Source: CAD feature listing. Evaluate the final solid. Frame: model axes, mm. A direction names the side the tool comes from. Give positions to 0.01 mm unless a question says otherwise; leave off trailing zeros. Order: outer loops, then holes, each group sorted by start corner. A loop starts at its lowest first (then second) coordinate and runs counter-clockwise, first axis right, second up.
1) Access query for faces 1 (the face through (96, 55, 61)), 2 (the face through (89, 100, 35)), 3 (the face through (13, 54, 10)), 4 (the face through (162, 45, 61)), 5 (the face through (100, 9, 70)). Directions: +Z, -Z, +X, -X, +Y, -Y. A direction counts if a zero-diameter tool reaches every point of the face in a straight line with its end or side. Return the directions, or none.
2) Draft query along X for faces 6 (the face through (156.15, 19.73, 60.14)), 7 (the face through (153.846, 57.509, 69.72)), 8 (the face through (15.3, 50.4, 20)), 9 (the face through (21.457, 49.54, 35.21)). Return one class per face: released by +X, released by -X, zero draft, split by the parting line, or undercut.
3) Section B-B, the plane x = 77.5. Return loops of the section in (y, z), plus the area to 3 significant figures.
4) Section A-A, the plane z = 28. Return loops of the section in (x, y), plus the area to 3 significant figures.
5) Section D-D, the plane z = 72.5. Return loops of the section in (x, y), plus the area to 3 significant figures.
6) Material intervals for line 1 (Y direction, x = 130, z = 80); line 2 (Y direction, x = 50, z = 20); line 3 (Y direction, x = 157, z = 59), sorted ascending.
7) Section C-C, the plane y = 22. Return loops of the section in (x, z).
8) First-contact query: P1, Ø6, axis at y = 44.5, z = 79, coming from the -X side; P2, Ø20, axis at x = 53, y = 46.5, coming from the +Z side; P3, Ø10.5, axis at x = 10, y = 61, coming from the +Z side; P4, Ø10, axis at x = 50.5, y = 51.5, coming from the +Z side. Flat tips, straight axial feed; report the tip coordinate or a pass-through.
```python
from build123d import *

# Parameters (mm, degrees)
SKETCH1_W                  = 180
SKETCH1_H                  = 100
BOSS_EXTRUDE2_DEPTH        = 70
CUT_EXTRUDE1_DEPTH         = 70
SKETCH3_R                  = 5
CUT_EXTRUDE2_DEPTH         = 70
SKETCH4_R                  = 5
CUT_EXTRUDE3_DEPTH         = 50
SKETCH5_R                  = 10
CUT_EXTRUDE4_DEPTH         = 106
SKETCH6_R                  = 15
CUT_EXTRUDE5_DEPTH         = 40
SKETCH8_R                  = 15
SKETCH8_R_2                = 12.5
BOSS_EXTRUDE3_DEPTH        = 40
SKETCH10_R                 = 12.5
BOSS_EXTRUDE4_DEPTH        = 65
F_25_0MM_DOWEL_HOLE2_D     = 25
F_25_0MM_DOWEL_HOLE2_DEPTH = 20
F_25_0MM_DOWEL_HOLE2_TIP   = 7.510757738
SKETCH12_R                 = 10
SKETCH12_R_2               = 12.5
CUT_EXTRUDE6_DEPTH         = 20
SKETCH13_R                 = 25
SKETCH13_R_2               = 12.5
BOSS_EXTRUDE5_DEPTH        = 40
SKETCH14_R                 = 20
SKETCH14_R_2               = 10
CUT_EXTRUDE7_DEPTH         = 20
BOSS_EXTRUDE10_DEPTH       = 30
BOSS_EXTRUDE13_DEPTH       = 30
CUT_EXTRUDE8_DEPTH         = 5


with BuildPart() as part:
    # Sketch1 → Boss-Extrude2 (new body)
    with BuildSketch(Plane.XY):
        with Locations((90, 50)):
            Rectangle(SKETCH1_W, SKETCH1_H)
    extrude(amount=BOSS_EXTRUDE2_DEPTH)

    # Sketch2 → Cut-Extrude1 (cut)
    with BuildSketch(Plane.XY.offset(70)):
        with BuildLine():
            Line((50, 100), (0, 100))
            Line((0, 100), (0, 50))
            ThreePointArc((0, 50), (14.644660941, 85.355339059), (50, 100))
        make_face()
        with BuildLine():
            ThreePointArc((50, 0), (14.644660941, 14.644660941), (0, 50))
            Line((0, 50), (0, 0))
            Line((0, 0), (50, 0))
        make_face()
        with BuildLine():
            Line((180, 0), (180, 50))
            ThreePointArc((180, 50), (165.355339059, 14.644660941), (130, 0))
            Line((130, 0), (180, 0))
        make_face()
        with BuildLine():
            Line((180, 100), (130, 100))
            ThreePointArc((130, 100), (165.355339059, 85.355339059), (180, 50))
            Line((180, 50), (180, 100))
        make_face()
    extrude(amount=-CUT_EXTRUDE1_DEPTH, mode=Mode.SUBTRACT)

    # Sketch3 → Cut-Extrude2 (cut)
    with BuildSketch(Plane.XY.offset(70)):
        with Locations((10, 50)):
            Circle(SKETCH3_R)
    extrude(amount=-CUT_EXTRUDE2_DEPTH, mode=Mode.SUBTRACT)

    # Sketch4 → Cut-Extrude3 (cut)
    with BuildSketch(Plane.XY.offset(70)):
        with BuildLine():
            ThreePointArc((10, 20), (21.458980338, 50), (10, 80))
            ThreePointArc((10, 80), (0, 50), (10, 20))
        make_face()
        with Locations((10, 50)):
            Circle(SKETCH4_R, mode=Mode.SUBTRACT)
    extrude(amount=-CUT_EXTRUDE3_DEPTH, mode=Mode.SUBTRACT)

    # Sketch5 → Cut-Extrude4 (cut)
    with BuildSketch(Plane.XY.offset(70)):
        with Locations((50, 50)):
            Circle(SKETCH5_R)
    extrude(amount=-CUT_EXTRUDE4_DEPTH, mode=Mode.SUBTRACT)

    # Sketch6 → Cut-Extrude5 (cut)
    with BuildSketch(Plane.XY.offset(70)):
        with Locations((130, 50)):
            Circle(SKETCH6_R)
    extrude(amount=-CUT_EXTRUDE5_DEPTH, mode=Mode.SUBTRACT)

    # Sketch8 → Boss-Extrude3 (add)
    with BuildSketch(Plane.XY.offset(70)):
        with Locations((130, 50)):
            Circle(SKETCH8_R)
        with Locations((130, 50)):
            Circle(SKETCH8_R_2, mode=Mode.SUBTRACT)
    extrude(amount=-BOSS_EXTRUDE3_DEPTH)

    # Sketch10 → Boss-Extrude4 (add)
    with BuildSketch(Plane.XY.offset(70)):
        with Locations((130, 50)):
            Circle(SKETCH10_R)
    extrude(amount=-BOSS_EXTRUDE4_DEPTH)

    # Ø25.0mm Dowel Hole2
    with Locations(Plane(origin=(130, 50, 70), x_dir=(1, 0, 0), z_dir=(0, 0, 1))):
        with Locations((0, 0)):
            Hole(F_25_0MM_DOWEL_HOLE2_D / 2, depth=F_25_0MM_DOWEL_HOLE2_DEPTH)
            with Locations((0, 0, -(F_25_0MM_DOWEL_HOLE2_DEPTH + F_25_0MM_DOWEL_HOLE2_TIP / 2))):  # 118° drill point
                Cone(0, F_25_0MM_DOWEL_HOLE2_D / 2, F_25_0MM_DOWEL_HOLE2_TIP, mode=Mode.SUBTRACT)

    # Sketch12 → Cut-Extrude6 (cut)
    with BuildSketch(Plane.XY.offset(70)):
        with BuildLine():
            ThreePointArc((130, 10), (170, 50), (130, 90))
            Line((130, 90), (20, 90))
            ThreePointArc((20, 90), (14.644660941, 85.355339059), (10, 80))
            ThreePointArc((10, 80), (21.458980338, 50), (10, 20))
            ThreePointArc((10, 20), (14.644660941, 14.644660941), (20, 10))
            Line((20, 10), (130, 10))
        make_face()
        with Locations((50, 50)):
            Circle(SKETCH12_R, mode=Mode.SUBTRACT)
        with Locations((130, 50)):
            Circle(SKETCH12_R_2, mode=Mode.SUBTRACT)
    extrude(amount=-CUT_EXTRUDE6_DEPTH, mode=Mode.SUBTRACT)

    # Sketch13 → Boss-Extrude5 (add)
    with BuildSketch(Plane.XY.offset(50)):
        with Locations((130, 50)):
            Circle(SKETCH13_R)
        with Locations((130, 50)):
            Circle(SKETCH13_R_2, mode=Mode.SUBTRACT)
    extrude(amount=BOSS_EXTRUDE5_DEPTH)

    # Sketch14 → Cut-Extrude7 (cut)
    with BuildSketch(Plane.XY.offset(50)):
        with Locations((50, 50)):
            Circle(SKETCH14_R)
        with Locations((50, 50)):
            Circle(SKETCH14_R_2, mode=Mode.SUBTRACT)
    extrude(amount=-CUT_EXTRUDE7_DEPTH, mode=Mode.SUBTRACT)

    # Sketch15 → Boss-Extrude10 (add)
    with BuildSketch(Plane.XY.offset(50)):
        with BuildLine():
            Line((105.505102572, 45), (105.505102572, 55))
            ThreePointArc((105.505102572, 55), (105, 50), (105.505102572, 45))
        make_face()
        with BuildLine():
            ThreePointArc((105.505102572, 45), (105, 50), (105.505102572, 55))
            Line((105.505102572, 55), (80.505102572, 55))
            Line((80.505102572, 55), (80.505102572, 45))
            Line((80.505102572, 45), (105.505102572, 45))
        make_face()
    extrude(amount=BOSS_EXTRUDE10_DEPTH)

    # Sketch16 → Boss-Extrude13 (add)
    with BuildSketch(Plane.XY.offset(50)):
        with BuildLine():
            Line((169.686269666, 55), (154.494897428, 55))
            ThreePointArc((154.494897428, 55), (155, 50), (154.494897428, 45))
            Line((154.494897428, 45), (169.686269666, 45))
            ThreePointArc((169.686269666, 45), (169.921490369, 47.495083498), (170, 50))
            ThreePointArc((170, 50), (169.921490369, 52.504916502), (169.686269666, 55))
        make_face()
    extrude(amount=BOSS_EXTRUDE13_DEPTH)

    # Sketch18 → Cut-Extrude8 (cut, symmetric)
    with BuildSketch(Plane(origin=(0, 50, 0), x_dir=(1, 0, 0), z_dir=(0, 1, 0))):
        Polygon((155.156999003, -80), (170.098617307, -70), (170.098617307, -80), align=None)
        Polygon((104.578940911, -80), (80.505102572, -50), (80.505102572, -80), align=None)
    extrude(amount=CUT_EXTRUDE8_DEPTH, both=True, mode=Mode.SUBTRACT)


solid = part.part
```
From the geometry:
1. face 1: +Z, -X
1. face 2: +Z, -Z, +X, -X, +Y
1. face 3: +Z, -Z
1. face 4: +Z
1. face 5: +Z, +X
2. face 6: undercut
2. face 7: undercut
2. face 8: zero draft
2. face 9: released by -X
3. outline: (0, 0) - (100, 0) - (100, 70) - (90, 70) - (90, 50) - (10, 50) - (10, 70) - (0, 70) - close
3. area: 5,400 mm2
4. outline: (10, 20) arc R50 ccw to (50, 0) - (130, 0) arc R50 ccw to (130, 100) - (50, 100) arc R50 ccw to (10, 80) arc R45 cw to start; hole circle Ø20 at (50, 50)
4. area: 14,700 mm2
5. outline: (98.56, 45) - (105.51, 45) arc R25 ccw to (154.49, 45) - (166.36, 45) - (166.36, 55) - (154.49, 55) arc R25 ccw to (105.51, 55) - (98.56, 55) - close; hole circle Ø25 at (130, 50)
5. area: 1,650 mm2
6. line 1: y = 25 to 37.5, 62.5 to 75
6. line 2: y = 0 to 40, 60 to 100
6. line 3: y = 7.92 to 20.49, 45 to 55, 79.51 to 92.08
7. outline: (8.58, 0) - (171.42, 0) - (171.42, 70) - (158.57, 70) - (158.57, 50) - (11.69, 50) - (11.69, 20) - (8.58, 20) - close
8. P1: stops at x = 101.4
8. P2: stops at z = 30
8. P3: stops at z = 20
8. P4: passes through
